The drawing under review shows one solid part. Ordinate dimensions are in mm from its lowest x, y, z. Round coordinates to 2 decimals unless told otherwise and drop trailing zeros. Order: outer loops, then holes, each group sorted by start corner. A loop starts at its lowest first (then second) coordinate and runs counter-clockwise, first axis right, second up. Notation, with made-up numbers: M 21,0.5 L 52,0.5 A28 cw 52,20.5 Z; hole C 24,83 d2. An arc over 180 degrees is marked long. Use a Markdown table: item, result.
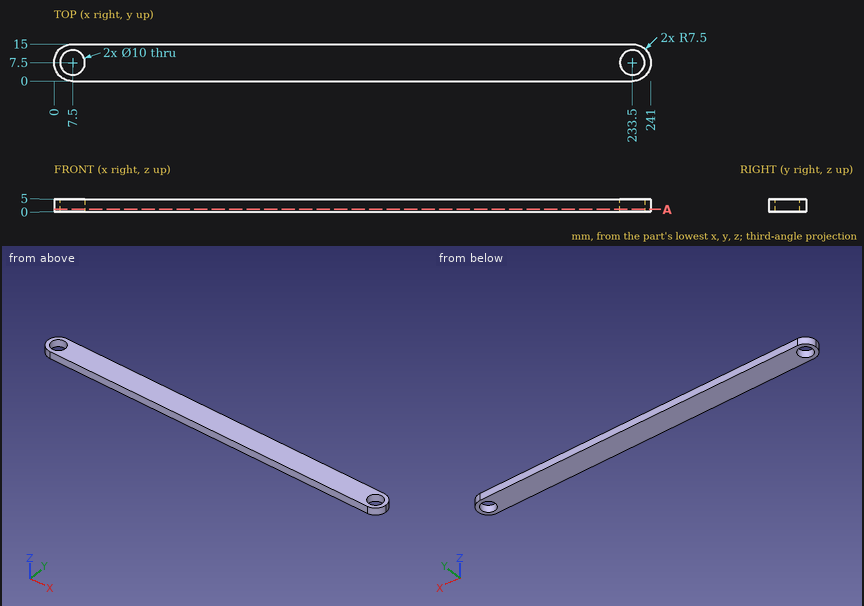
Q1. Wall thickness on line 1 along X through (y, z) = (7.75, 4.75); line 2 along Y through (x, z) = (233.5, 1.6); line 3 along X through (y, z) = (5.25, 1.7): over which ranges is each line inside the solid? List them lowest first. Write a range as [from, to].
Determined:
| item | result |
|---|---|
| line 1 | x = [0, 2.51], [12.49, 228.51], [238.49, 241] |
| line 2 | y = [0, 2.5], [12.5, 15] |
| line 3 | x = [0.35, 3.03], [11.97, 229.03], [237.97, 240.65] |
Q2. Clearance check with flat-ended pins moving along their axes: pin 1 (1 mm diameter, centred on y = 4, z = 1.5, fed in from +X); pin 2 (6 mm diameter, centred on x = 233.5, y = 7.5, fed in from -Z). State where each tip first meets the part, or that it passes through.
Determined:
| item | result |
|---|---|
| pin 1 | stops at x = 240.37 |
| pin 2 | passes through |
Q3. Add section A-A (z = 0.85). Write out the cut boundary in (x, y), then the cut area to 3 significant figures.
Determined:
| item | result |
|---|---|
| outline | M 7.5,0 L 233.5,0 A7.5 ccw 233.5,15 L 7.5,15 A7.5 ccw Z; hole C 7.5,7.5 d10; hole C 233.5,7.5 d10 |
| area | 3,410 mm^2 |
